Here's how the part is built. I have some questions about the finished solid (model axes, mm). A direction names the side the tool comes from. Give positions to 0.01 mm unless a question says otherwise; leave off trailing zeros. Write each loop counter-clockwise with the first axis right and the second up, starting at its lowest first coordinate (ties: lowest second). Pieces come first, ordered by that corner, then holes. Notation, with made-up numbers: (-31.75, 52) - (24.25, 52) arc R12 ccw to (24.25, 57) - close; hole circle Ø7 at (76.5, 45.25). An arc over 180 degrees is marked (long way). One line per item, written item: value. Start each with the question number.
1) On a 3-axis mill with a long thin cutter (end or side, diameter ignored), from which of +Z, -Z, +X, -X, +Y, -Y can I reach the whole of each face in a straight line? I mean faces 1 (the flat face through (2, 73, 75.749)), 2 (the flat face through (2, 76, 50.387)), 3 (the flat face through (-32.18, 73, 37)), 4 (the flat face through (-12.998, 58, 100)). Say none if no direction works.
2) Please list where these lines run through material, in increasing order: L1, parallel to Y at x = 36, z = 80.5; L2, parallel to X at y = 67.5, z = 66; L3, parallel to Y at x = 20.5, z = 102.5. Write a range as [from, to].
3) Imagine slicing it at B-B on x = -20.5. Write out the boundary of the cut face in (y, z).
4) We'd pull the mould along X, two halves only. Please class faces 5 (the flat face through (37.888, 73, 38)), 6 (the flat face through (3, 58, 110.77)), 7 (the flat face through (0, -56.03, 63)): +X half, -X half, draft (parallel to the pull), parting line (faces both ways), or undercut.
5) Imagine slicing it at D-D on z = 9. Write out the boundary of the cut face in (x, y).
6) Imagine slicing it at A-A on z = 96. Write out the boundary of the cut face in (x, y), plus the area to 3 significant figures.
7) Imagine slicing it at C-C on y = 75. Write out the boundary of the cut face in (x, z), plus the area to 3 significant figures.
8) I'm going to push flat-ended pins straight in: P1, Ø6, axis at y = 78, z = 34.5, coming from the +X side; P2, Ø1, axis at x = 42, z = 21, coming from the +Y side; P3, Ø7.5, axis at x = -2.5, y = 77.5, coming from the +Z side. Where does each tip first touch, or does it pass through?
from build123d import *

# Parameters (mm, degrees)
F0_W      = 105.8345548809
F0_H      = 111.5989610553
F1_DEPTH  = 127
F2_W      = 105.8345548809
F2_H      = 127
F2_W_2    = 22.996397689
F2_H_2    = 22.2293362021
F3_DEPTH  = 5.08
F4_W      = 26.9106691703
F4_H      = 50.3869839013
F5_DEPTH  = 5.08
F7_DEPTH  = 25.4
F8_W      = 22.5071115419
F8_H      = 21.3920027018
F9_DEPTH  = 5.08
F10_W     = 22.0178281888
F10_H     = 21.4731246233
F11_DEPTH = 5.08
F12_W     = 10.2898292243
F12_H     = 61.8074573576
F13_DEPTH = 5.08


with BuildPart() as f1:
    # F0 (on Top) → F1 (new body)
    with BuildSketch(Plane.XY):
        with Locations((0.5764421076, -0.230576843)):
            Rectangle(F0_W, F0_H)
    extrude(amount=F1_DEPTH)

    # F2 (on face) → F3 (join)
    with BuildSketch(Plane(origin=(0, 55.5689036846, 0), x_dir=(-1, 0, 0), z_dir=(0, 1, 0))):
        with Locations((-0.5764421076, 63.5)):
            Rectangle(F2_W, F2_H)
        with Locations((-31.7689729854, 99.5473898947)):
            Rectangle(F2_W_2, F2_H_2, mode=Mode.SUBTRACT)
    extrude(amount=F3_DEPTH)

    # F4 (on face) → F5 (join)
    with BuildSketch(Plane(origin=(0, 60.6489036846, 0), x_dir=(-1, 0, 0), z_dir=(0, 1, 0))):
        with Locations((-1.4360728674, 25.1934919506)):
            Rectangle(F4_W, F4_H)
    extrude(amount=F5_DEPTH)

    # F6 (on face) → F7 (join)
    with BuildSketch(Plane(origin=(0, 60.6489036846, 0), x_dir=(-1, 0, 0), z_dir=(0, 1, 0))):
        Polygon((-37.8878116608, 0), (-29.5699629933, 0), (-29.5699629933, 55.8542273939), (22.2942437977, 55.8542273939), (22.2942437977, 0), (32.1800485253, 0), (32.1800485253, 75.7494047284), (-37.8878116608, 75.7494047284), align=None)
        Polygon((-29.5699629933, 55.8542273939), (-29.5699629933, 0), (-14.8914074525, 0), (-14.8914074525, 50.3869839013), (12.0192617178, 50.3869839013), (12.0192617178, 0), (22.2942437977, 0), (22.2942437977, 55.8542273939), align=None)
    extrude(amount=F7_DEPTH)

    # F8 (on face) → F9 (cut)
    with BuildSketch(Plane(origin=(0, 60.6489036846, 0), x_dir=(-1, 0, 0), z_dir=(0, 1, 0))):
        with Locations((-3.1485739164, 100.074402988)):
            Rectangle(F8_W, F8_H)
    extrude(amount=-F9_DEPTH, mode=Mode.SUBTRACT)

    # F10 (on face) → F11 (cut)
    with BuildSketch(Plane(origin=(0, 60.6489036846, 0), x_dir=(-1, 0, 0), z_dir=(0, 1, 0))):
        with Locations((24.006747175, 100.1149639487)):
            Rectangle(F10_W, F10_H)
    extrude(amount=-F11_DEPTH, mode=Mode.SUBTRACT)

    # F12 (on face) → F13 (cut)
    with BuildSketch(Plane(origin=(0, 86.0489036846, 0), x_dir=(-1, 0, 0), z_dir=(0, 1, 0))):
        with Locations((-27.1603707224, 30.9037286788)):
            Rectangle(F12_W, F12_H)
    extrude(amount=-F13_DEPTH, mode=Mode.SUBTRACT)


solid = f1.part
Numbers:
1. face 1: +Z, +X, -X, +Y
1. face 2: -Z, +Y
1. face 3: +Z, -Z, -X, +Y
1. face 4: +Y
2. L1: [-56.03, 60.65]
2. L2: [-32.18, 37.89]
2. L3: [-56.03, 55.57]
3. outline: (-56.03, 0) - (86.05, 0) - (86.05, 75.75) - (60.65, 75.75) - (60.65, 89.38) - (55.57, 89.38) - (55.57, 110.85) - (60.65, 110.85) - (60.65, 127) - (-56.03, 127) - close
4. face 5: +X half
4. face 6: undercut
4. face 7: draft
5. outline: (-52.34, -56.03) - (53.49, -56.03) - (53.49, 60.65) - (37.89, 60.65) - (37.89, 86.05) - (32.31, 86.05) - (32.31, 80.97) - (22.02, 80.97) - (22.02, 86.05) - (14.89, 86.05) - (14.89, 65.73) - (-12.02, 65.73) - (-12.02, 86.05) - (-32.18, 86.05) - (-32.18, 60.65) - (-52.34, 60.65) - close
6. outline: (-52.34, -56.03) - (53.49, -56.03) - (53.49, 60.65) - (43.27, 60.65) - (43.27, 55.57) - (20.27, 55.57) - (20.27, 60.65) - (14.4, 60.65) - (14.4, 55.57) - (-8.1, 55.57) - (-8.1, 60.65) - (-13, 60.65) - (-13, 55.57) - (-35.02, 55.57) - (-35.02, 60.65) - (-52.34, 60.65) - close
6. area: 12,000 mm^2
7. outline: (-32.18, 0) - (-12.02, 0) - (-12.02, 50.39) - (14.89, 50.39) - (14.89, 0) - (37.89, 0) - (37.89, 75.75) - (-32.18, 75.75) - close
7. area: 3,950 mm^2
8. P1: x = 37.89
8. P2: y = 60.65
8. P3: z = 75.75
